Source: CAD feature listing. Evaluate the final solid. Frame: model axes, mm. Face numbers are marked on the shaded views. A direction names the side the tool comes from. Coordinates: 2 decimals unless noted, no trailing zeros. Loops run counter-clockwise (first coordinate to the right, second up) from the corner with the lowest first, then second, coordinate; pieces in that order, holes last. Notation, with made-up numbers: (-38.5, -37) - (-15.5, -37) arc R26 cw to (-15.5, -18) - close; hole circle Ø6 at (48, 72.25). An arc over 180 degrees is marked (long way). Write item = value, one per line. Start each with the question number.
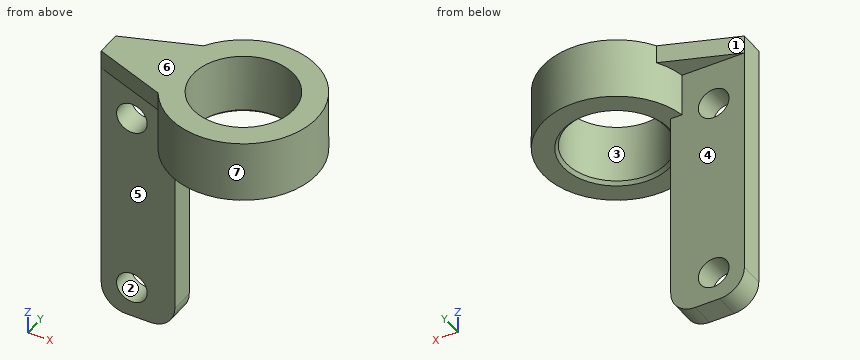
from build123d import *

# Parameters (mm, degrees)
SKETCH_R     = 12
SKETCH_R_2   = 8.2
PAD_DEPTH    = 10
SKETCH001_W  = 12
SKETCH001_H  = 4
PAD001_DEPTH = 45
SKETCH003_R  = 2.5
POCKET_DEPTH = 5
PAD002_DEPTH = 3
FILLET_R     = 4
CHAMFER_SIZE = 0.5


with BuildPart() as part:
    # Sketch → Pad (new body)
    with BuildSketch(Plane.XY):
        Circle(SKETCH_R)
        Circle(SKETCH_R_2, mode=Mode.SUBTRACT)
    extrude(amount=PAD_DEPTH)

    # Sketch001 (on Face4 of Pad) → Pad001 (join)
    with BuildSketch(Plane.XY.offset(10)):
        with Locations((-16, 0)):
            Rectangle(SKETCH001_W, SKETCH001_H)
    extrude(amount=-PAD001_DEPTH)

    # Sketch003 (on Face6 of Pad001) → Pocket (cut)
    with BuildSketch(Plane.XZ.offset(2)):
        with Locations((-17, 0)):
            Circle(SKETCH003_R)
        with Locations((-17, -30)):
            Circle(SKETCH003_R)
    extrude(amount=-POCKET_DEPTH, mode=Mode.SUBTRACT)

    # Sketch005 (on Face10 of Pocket) → Pad002 (join)
    with BuildSketch(Plane.XY.offset(10)):
        Polygon((-22, 2), (-9.44483, 6.578776), (-9.44483, -6.578776), (-22, -2), align=None)
    extrude(amount=-PAD002_DEPTH)

    # Fillet
    fillet_edges = [part.edges().sort_by_distance(p)[0] for p in [
        (-22, 0, -35),
        (-10, 0, -35),
    ]]
    fillet(fillet_edges, radius=FILLET_R)

    # Chamfer
    chamfer_edges = [part.edges().sort_by_distance(p)[0] for p in [
        (-8.2, 0, 0),
    ]]
    chamfer(chamfer_edges, length=CHAMFER_SIZE)


solid = part.part
Item 1: Cut plane A-A (y = 0). Return the cut outline in (x, z).
Item 2: Draft query along Y for the marked faces 1, 2 and 3. Return one class per face: released by +Y, released by -Y, zero draft, split by the parting line, or undercut.
Item 3: Cut plane D-D (z = 7.5). Return the cut outline in (x, y).
Item 4: Material intervals for L1, parallel to Z at x = -17, y = 1.05; L2, parallel to Y at x = 0, z = 6; L3, parallel to Z at x = 8.5, y = -7.5, sorted ascending. Write a range as [from, to].
Item 5: First-contact query: pin 1 (1 mm diameter, centred on y = -4, z = -21.5, fed in from +X); pin 2 (2 mm diameter, centred on x = -17.5, y = -3.5, fed in from -Z); pin 3 (3.5 mm diameter, centred on x = -16, z = -18.5, fed in from +Y); pin 4 (8 mm diameter, centred on x = -0.5, y = 5.5, fed in from -Z). Flat tips, straight axial feed; report the tip coordinate or a pass-through.
Item 6: Reachability of the marked faces 4, 5, 6 and 7 from +Z, -Z, +X, -X, +Y, -Y: full face, straight path, thin tool, end or side. Return the list, or none.
Item 7: Cut plane B-B (z = -30). Return the cut outline in (x, y).
Item 8: Cut plane C-C (x = 0). Return the cut outline in (y, z), then the cut area to 4 significant figures.
Responses:
q1.outline = (-22, -31) arc R4 ccw to (-18, -35) - (-14, -35) arc R4 ccw to (-10, -31) - (-10, 0) - (-8.7, 0) - (-8.2, 0.5) - (-8.2, 10) - (-22, 10) - close; (8.2, 0.5) - (8.7, 0) - (12, 0) - (12, 10) - (8.2, 10) - close; hole circle Ø5 at (-17, -30); hole circle Ø5 at (-17, 0)
q2.face_1 = released by +Y
q2.face_2 = zero draft
q2.face_3 = undercut
q3.outline = (-22, -2) - (-10.21, -6.3) arc R12 ccw (long way) to (-10.21, 6.3) - (-22, 2) - close; hole circle Ø16.4 at (0, 0)
q4.L1 = [-35, -32.5], [-27.5, -2.5], [2.5, 10]
q4.L2 = [-12, -8.2], [8.2, 12]
q4.L3 = [0, 10]
q5.pin_1 = through
q5.pin_2 = 7
q5.pin_3 = 2
q5.pin_4 = 0
q6.face_4 = -Z, -X, +Y
q6.face_5 = -Z, -X, -Y
q6.face_6 = +Z, +X, -X, +Y, -Y
q6.face_7 = -Z
q7.outline = (-22, -2) - (-19.5, -2) - (-19.5, 2) - (-22, 2) - close; (-14.5, -2) - (-10, -2) - (-10, 2) - (-14.5, 2) - close
q8.outline = (-12, 0) - (-8.7, 0) - (-8.2, 0.5) - (-8.2, 10) - (-12, 10) - close; (8.2, 0.5) - (8.7, 0) - (12, 0) - (12, 10) - (8.2, 10) - close
q8.area = 75.75 mm2
